Read the model definition and answer for the solid it produces. Units are mm, in the model's axes. Face numbers are marked on the shaded views. A direction names the side the tool comes from. Coordinates: 2 decimals unless noted, no trailing zeros. Order: outer loops, then holes, each group sorted by start corner. A loop starts at its lowest first (then second) coordinate and runs counter-clockwise, first axis right, second up. Notation, with made-up numbers: M 1.5,65 L 15.5,65 A15 ccw 15.5,77 Z; hole C 25,67.5 d6. An arc over 180 degrees is marked long. Put each result on its own line as item: value.
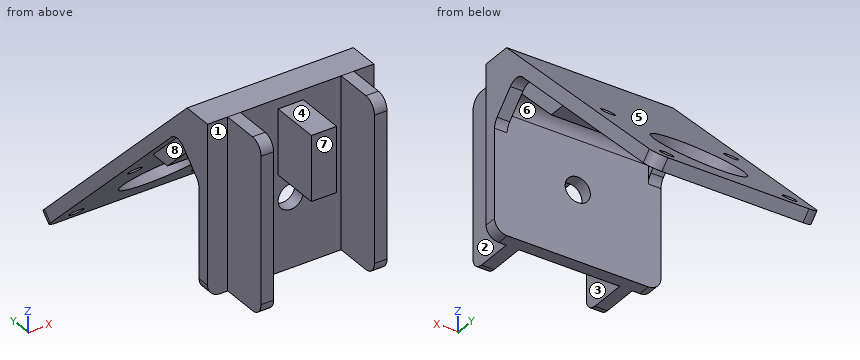
Autodesk Inventor part; units mm, degrees
ref_plane "YZ Plane" through (0, 0, 0) normal (1, 0, 0) x (0, 1, 0)
ref_plane "XZ Plane" through (0, 0, 0) normal (0, 1, 0) x (-1, 0, 0)
ref_plane "XY Plane" through (0, 0, 0) normal (0, 0, 1) x (1, 0, 0)
sketch "Sketch1" plane through (0, 0, 0) normal (0, 1, 0) x (-1, 0, 0)
  line L0 (9.3294, -16.9333) -> (-32.5806, -16.9333)
  line L1 (-32.5806, -16.9333) -> (-32.5806, 33.8667)
  line L2 (-32.5806, 33.8667) -> (9.3294, 33.8667)
  line L3 (9.3294, 33.8667) -> (9.3294, -16.9333)
  point P0 (0, 0)
  dimension "d0" = 50.8
  dimension "d1" = 41.91
extrude "Extrusion1" add sketch "Sketch1" along normal blind 3.175
chamfer "Chamfer1" distance 3.175 angle 45 1 edges at (11.6256, 3.175, 33.8667)
sketch "Sketch9" plane through (32.5806, 0, -16.9333) normal (1, 0, 0) x (0, 0, -1)
  line L0 (-47.625, 3.175) -> (0, 3.175)
  line L1 (-11.631, 34.6788) -> (-43.1349, 3.175)
  line L2 (-13.8761, 36.9239) -> (-11.631, 34.6788)
  line L3 (-34.9797, 11.3302) -> (-26.8245, 3.175)
  point P0 (-16.9333, 0)
  dimension "d15" = 33.02
extrude "Extrusion4" add sketch "Sketch9" against normal blind 3.175
sketch "Sketch10" plane through (-9.3294, 0, -16.9333) normal (-1, 0, 0) x (0, 0, 1)
  line L0 (0, 3.175) -> (47.625, 3.175)
  line L1 (13.8761, 36.9239) -> (11.631, 34.6788)
  line L2 (43.1349, 3.175) -> (11.631, 34.6788)
  line L3 (34.9797, 11.3302) -> (26.8245, 3.175)
  point P0 (16.9333, 0)
  dimension "d18" = 33.02
extrude "Extrusion5" add sketch "Sketch10" against normal blind 3.175
fillet "Fillet3" radius 3.175 2 edges at (-7.7419, 3.175, 9.8912) (30.9931, 3.175, 9.8912)
fillet "Fillet4" radius 3.175 2 edges at (-9.3294, 1.5875, -16.9333) (32.5806, 1.5875, -16.9333)
sketch "Sketch11" plane through (0, 0, 0) normal (0, -1, 0) x (1, 0, 0)
  line L0 (-9.3294, 26.2015) -> (32.5806, 26.2015)
  line L1 (-9.3294, 33.8667) -> (-9.3294, -13.7583)
  line L2 (-6.1544, -16.9333) -> (29.4056, -16.9333)
  line L3 (32.5806, -13.7583) -> (32.5806, 33.8667)
  line L4 (11.6256, 26.2015) -> (11.6256, -16.9333)
  line L5 (-9.3294, 0.8015) -> (32.5806, 0.8015)
  circle A0 centre (11.6256, 0.8015) radius 3.175
  point P0 (0, 0)
  dimension "d24" = 20.955
  dimension "d25" = 25.4
  dimension "d26" = 6.35
extrude "Extrusion9" cut sketch "Sketch11" against normal blind 12.446 contours A0 L5 L4 | L4 L5 A0 | L5 L4 A0 | L5 A0 L4
sketch "Sketch19" plane through (0, 0, 0) normal (0, -1, 0) x (1, 0, 0)
  circle A0 centre (11.6256, 0.8015) radius 3.175
  circle A1 centre (11.6256, -9.3585) radius 3.175
  point P0 (0, 0)
  dimension "d44" = 6.35
  dimension "d45" = 10.16
  dimension "d46" = 0
extrude "Extrusion10" add sketch "Sketch19" along normal blind 12.446 contours A1
sketch "Sketch20" plane through (0, 0, 0) normal (0, -1, 0) x (1, 0, 0)
  circle A0 centre (11.6256, 0.8015) radius 3.175
  circle A1 centre (11.6256, 10.9615) radius 3.175
  point P0 (0, 0)
  dimension "d49" = 6.35
  dimension "d50" = 10.16
  dimension "d51" = 0
extrude "Extrusion11" add sketch "Sketch20" along normal blind 12.446 contours A1
sketch "Sketch24" plane through (0, 0, 0) normal (0, -1, 0) x (1, 0, 0)
  circle A0 centre (11.6256, 0.8015) radius 3.175
  line L0 (-9.3294, 26.2015) -> (32.5806, 26.2015)
  line L1 (-6.1544, -16.9333) -> (29.4056, -16.9333)
  line L2 (24.3256, 26.2015) -> (24.3256, -16.9333)
  line L3 (24.3256, 26.2015) -> (27.5006, 26.2015)
  line L4 (27.5006, 26.2015) -> (27.5006, -16.9333)
  line L5 (27.5006, -16.9333) -> (24.3256, -16.9333)
  line L6 (24.3256, -16.9333) -> (24.3256, 26.2015)
  point P0 (0, 0)
  dimension "d64" = 12.7
  dimension "d65" = 3.175
extrude "Extrusion14" add sketch "Sketch24" along normal blind 12.446 contours L0 L4 L1 L2
sketch "Sketch25" plane through (0, 0, 0) normal (0, -1, 0) x (1, 0, 0)
  circle A0 centre (11.6256, 0.8015) radius 3.175
  line L0 (-9.3294, 26.2015) -> (24.3256, 26.2015)
  line L1 (-6.1544, -16.9333) -> (24.3256, -16.9333)
  line L2 (-1.0744, 26.2015) -> (-1.0744, -16.9333)
  line L3 (-1.0744, -16.9333) -> (-4.2494, -16.9333)
  line L4 (-4.2494, -16.9333) -> (-4.2494, 26.2015)
  line L5 (-4.2494, 26.2015) -> (-1.0744, 26.2015)
  line L6 (-1.0744, 26.2015) -> (-1.0744, -16.9333)
  point P0 (0, 0)
  dimension "d68" = 12.7
  dimension "d69" = 3.175
extrude "Extrusion15" add sketch "Sketch25" along normal blind 12.446 contours L0 L2 L1 L4
fillet "Fillet8" radius 3.175 4 edges at (25.9131, -12.446, 26.2015) (25.9131, -12.446, -16.9333) (-2.6619, -12.446, -16.9333) (-2.6619, -12.446, 26.2015)
sketch "Sketch28" plane through (-9.3294, 3.175, 30.6917) normal (0, 0.7071068, 0.7071068) x (1, 0, 0)
  line L0 (41.91, -4.4901) -> (41.91, 0)
  line L1 (41.91, 0) -> (0, 0)
  line L2 (0, 0) -> (0, -4.4901)
  line L3 (41.91, -4.4901) -> (0, -4.4901)
  line L4 (0, -4.4901) -> (41.91, -4.4901)
  line L5 (41.91, -4.4901) -> (41.91, 85.0449)
  line L6 (41.91, 85.0449) -> (0, 85.0449)
  line L7 (0, 85.0449) -> (0, -4.4901)
  point P0 (9.3294, 19.4572)
  dimension "d75" = 41.91
  dimension "d76" = 89.535
extrude "Extrusion16" add sketch "Sketch28" against normal blind 3.175 contours L1 L7 L6 L5
sketch "Sketch29" plane through (-9.3294, 0, 33.8667) normal (0, 0.7071068, 0.7071068) x (1, 0, 0)
  line L0 (41.91, 89.535) -> (0, 89.535)
  line L1 (0, 89.535) -> (0, 0)
  circle A0 centre (20.955, 68.58) radius 11.1125
  point P0 (9.3294, 23.9473)
  dimension "d79" = 22.225
  dimension "d80" = 20.955
  dimension "d81" = 20.955
extrude "Extrusion17" cut sketch "Sketch29" against normal blind 3.175
sketch "Sketch30" plane through (-9.3294, 0, 33.8667) normal (0, 0.7071068, 0.7071068) x (1, 0, 0)
  circle A0 centre (20.955, 68.58) radius 11.1125
  circle A1 centre (5.461, 84.074) radius 1.7272
  point P0 (9.3294, 23.9473)
  dimension "d84" = 3.4544
  dimension "d85" = 15.494
  dimension "d86" = 15.494
extrude "Extrusion18" cut sketch "Sketch30" against normal blind 3.175 contours A1
sketch "Sketch31" plane through (-9.3294, 0, 33.8667) normal (0, 0.7071068, 0.7071068) x (1, 0, 0)
  circle A0 centre (5.461, 84.074) radius 1.7272
  circle A1 centre (20.955, 68.58) radius 11.1125
  circle A2 centre (5.461, 53.086) radius 1.7272
  point P0 (9.3294, 23.9473)
  dimension "d89" = 3.4544
  dimension "d90" = 3.4544
  dimension "d91" = 15.494
  dimension "d92" = 15.494
extrude "Extrusion19" cut sketch "Sketch31" against normal blind 3.175 contours A2
sketch "Sketch32" plane through (-9.3294, 0, 33.8667) normal (0, 0.7071068, 0.7071068) x (1, 0, 0)
  circle A0 centre (20.955, 68.58) radius 11.1125
  circle A1 centre (36.449, 84.074) radius 1.7272
  point P0 (9.3294, 23.9473)
  dimension "d95" = 3.4544
  dimension "d96" = 15.494
  dimension "d97" = 15.494
extrude "Extrusion20" cut sketch "Sketch32" against normal blind 3.175 contours A1
sketch "Sketch33" plane through (-9.3294, 0, 33.8667) normal (0, 0.7071068, 0.7071068) x (1, 0, 0)
  circle A0 centre (20.955, 68.58) radius 11.1125
  circle A1 centre (36.449, 53.086) radius 1.7272
  point P0 (9.3294, 23.9473)
  dimension "d100" = 3.4544
  dimension "d101" = 15.494
  dimension "d102" = 15.494
extrude "Extrusion21" cut sketch "Sketch33" against normal blind 3.175 contours A1
fillet "Fillet9" radius 3.175 2 edges at (-9.3294, 62.1883, -30.5667) (32.5806, 62.1883, -30.5667)
fillet "Fillet10" radius 3.175 2 edges at (30.9931, 11.3302, 18.0464) (-7.7419, 11.3302, 18.0464)
sketch "Sketch37" plane through (11.6256, -12.446, 10.9615) normal (0, -1, 0) x (1, 0, 0)
  line L0 (-15.875, 12.065) -> (-15.875, -24.7199)
  line L1 (-12.7, -24.7199) -> (-12.7, 12.065)
  circle A0 centre (0, 0) radius 3.175
  line L2 (-3.175, 0) -> (3.175, 0)
  line L3 (3.175, 0) -> (3.175, 12.7)
  line L4 (3.175, 12.7) -> (-3.175, 12.7)
  line L5 (-3.175, 12.7) -> (-3.175, 0)
  point P0 (-11.6256, -10.9615)
  dimension "d111" = 3.175
  dimension "d112" = 6.35
  dimension "d113" = 12.7
extrude "Extrusion22" add sketch "Sketch37" against normal blind 12.954 contours L2 A0 | A0 L5 L4 L3 picked at (0.7922, 0.7018)
sketch "Sketch38" plane through (0, -12.446, 0) normal (0, -1, 0) x (1, 0, 0)
  line L0 (14.8006, 10.9615) -> (14.8006, 23.6615)
  line L1 (14.8006, 16.2386) -> (8.4506, 16.2386)
  line L2 (8.4506, 16.2386) -> (8.4506, 7.2793)
  line L3 (8.4506, 7.2793) -> (14.8006, 7.2793)
  line L4 (14.8006, 7.2793) -> (14.8006, 16.2386)
  point P0 (0, 0)
  dimension "d116" = 6.35
extrude "Extrusion23" add sketch "Sketch38" against normal blind 12.954
sketch "Sketch39" plane through (11.6256, -12.446, -9.3585) normal (0, -1, 0) x (1, 0, 0)
  line L0 (3.175, -3.175) -> (-3.175, -3.175)
  line L1 (-3.175, -3.175) -> (-3.175, 3.175)
  line L2 (-3.175, 3.175) -> (3.175, 3.175)
  line L3 (3.175, 3.175) -> (3.175, -3.175)
  point P0 (-11.6256, 9.3585)
  dimension "d119" = 6.35
  dimension "d120" = 6.35
extrude "Extrusion24" add sketch "Sketch39" against normal blind 12.954
fillet "Fillet12" radius 3.175 1 edges at (14.8006, -6.223, -12.5335)
fillet "Fillet13" radius 3.175 1 edges at (8.4506, -6.223, -12.5335)
sketch "Sketch44" plane through (32.5806, 0, 33.8667) normal (1, 0, 0) x (0, 0, -1)
  line L0 (7.6651, 0) -> (7.6651, 7.6651)
  line L1 (61.0657, 61.0657) -> (0, 0)
  line L2 (0, 0) -> (7.6651, 0)
  line L3 (47.625, 0) -> (0, 0)
  line L4 (7.6651, 7.6651) -> (0, 0)
  point P0 (33.8667, 0)
extrude "Extrusion25" cut sketch "Sketch44" against normal blind 76.2
sketch "Sketch45" plane through (-9.3294, 0.9299, 28.4466) normal (0, -0.7071068, -0.7071068) x (-1, 0, 0)
  line L0 (-38.735, 3.175) -> (-3.175, 3.175)
  line L1 (-3.175, 3.175) -> (-3.175, 34.1687)
  line L2 (-3.175, 34.1687) -> (-38.735, 34.1687)
  line L3 (-38.735, 34.1687) -> (-38.735, 3.175)
  line L4 (-3.175, 3.175) -> (-3.175, 17.8832)
  circle A0 centre (-36.449, 48.5959) radius 1.7272
  point P0 (-9.3294, 19.4572)
  dimension "d129" = 0
  dimension "d130" = 12.7
extrude "Extrusion26" add sketch "Sketch45" along normal blind 3.81 contours L3 L2 L1 L0
chamfer "Chamfer2" distance 3.81 angle 45 1 edges at (11.6256, 22.3968, 1.5916)
fillet "Fillet14" radius 3.175 1 edges at (11.6256, 3.175, 20.8134)
sketch "Sketch47" plane through (0, -12.446, 0) normal (0, -1, 0) x (1, 0, 0)
  line L0 (14.8006, -6.1835) -> (8.4506, -6.1835)
  line L1 (8.4506, -6.1835) -> (8.4506, -12.6132)
  line L2 (8.4506, -12.6132) -> (14.8006, -12.6132)
  line L3 (14.8006, -12.6132) -> (14.8006, -6.1835)
  point P0 (0, 0)
extrude "Extrusion27" cut sketch "Sketch47" against normal blind 12.446
properties part number "slider"
Q1. Given pin 1 (6 mm diameter, centred on y = 17.5, z = 9.5, fed in from +X); pin 2 (10 mm diameter, centred on x = 14.5, y = 0, fed in from -Z); pin 3 (5 mm diameter, centred on x = 12, y = 23, fed in from -Z); pin 4 (3 mm diameter, centred on x = 12.5, y = -9, fed in from -Z), each flat-ended and moving along its own axis, determine where each tip first touches the part or whether it passes through.
Answers below:
pin 1: stops at x = 32.58
pin 2: stops at z = -16.93
pin 3: stops at z = 3.88
pin 4: stops at z = 7.28
Q2. Find section B-B on x = 11. Give the number of separate pieces and of enclosed holes in the cut face, plus the area to 3 significant figures.
Answers below:
separate pieces: 3
enclosed holes: 0
area: 622 mm^2
Q3. A tool of negligible diameter and unlimited length cuts with its end or side. For the marked faces 1, 2, 3 and 4, from which of +Z, -Z, +X, -X, +Y, -Y can it reach the whole face along a straight path? Write none if from no direction.
Answers below:
face 1: +Z, -Z, -X, -Y
face 2: +Z, -Z, +X, -Y
face 3: +Z, -Z, -Y
face 4: +Z, -Y
Q4. Consider line 1 along X through (y, z) = (-1, 12); line 2 along Y through (x, z) = (10, -4) (3 decimals); line 3 along Y through (x, z) = (0, 10) (3 decimals). Determine where each line is inside the solid, lowest interval first.
Answers below:
line 1: x = -4.25 to -1.07, 8.45 to 14.8, 24.33 to 27.5
line 2: y = 0 to 3.175, 33.377 to 37.867
line 3: y = 0 to 3.175, 13.988 to 23.867
Q5. For a pull along Y with two mould halves and no side action, classify the marked faces 5, 6, 7 and 8 as +Y half, -Y half, draft (parallel to the pull), parting line (faces both ways), or undercut.
Answers below:
face 5: +Y half
face 6: undercut
face 7: -Y half
face 8: undercut
Q6. Find section C-C on y = 11. Write down the section's boundary in (x, z), plus the area to 3 significant figures.
Answers below:
outline: M -9.33,16.71 L -6.15,16.71 L -6.15,12.99 L 29.41,12.99 L 29.41,16.71 L 32.58,16.71 L 32.58,22.87 L -9.33,22.87 Z
area: 390 mm^2
